```python
from build123d import *

# Parameters (mm, degrees)
SKETCH2_W              = 90
SKETCH2_H              = 90
BOSS_EXTRUDE1_DEPTH    = 300
SKETCH3_W              = 45
SKETCH3_H              = 255
CUT_EXTRUDE1_DEPTH     = 317.425346646
SKETCH4_R              = 25
CRANK_SHAFT_HOLE_DEPTH = 90
SKETCH5_R              = 13
CUT_EXTRUDE3_DEPTH     = 90
CHAMFER1_SIZE          = 3
SKETCH6_R              = 17.5
BOSS_EXTRUDE2_DEPTH    = 30


with BuildPart() as part:
    # Sketch2 → Boss-Extrude1 (new body)
    with BuildSketch(Plane(origin=(0, 0, 0), x_dir=(1, 0, 0), z_dir=(0, 1, 0))):
        Rectangle(SKETCH2_W, SKETCH2_H)
    extrude(amount=BOSS_EXTRUDE1_DEPTH)

    # Sketch3 → Cut-Extrude1 (cut, through all)
    with BuildSketch(Plane(origin=(45, 0, 0), x_dir=(0, 0, -1), z_dir=(1, 0, 0))):
        with Locations((0, 150)):
            Rectangle(SKETCH3_W, SKETCH3_H)
    extrude(amount=-CUT_EXTRUDE1_DEPTH, mode=Mode.SUBTRACT)

    # Sketch4 → Crank shaft hole (cut)
    with BuildSketch(Plane.XY.offset(45)):
        with Locations((0, 170.5)):
            Circle(SKETCH4_R)
    extrude(amount=-CRANK_SHAFT_HOLE_DEPTH, mode=Mode.SUBTRACT)

    # Sketch5 → Cut-Extrude3 (cut)
    with BuildSketch(Plane.XY.offset(45)):
        with Locations((0, 45)):
            Circle(SKETCH5_R)
    extrude(amount=-CUT_EXTRUDE3_DEPTH, mode=Mode.SUBTRACT)

    # Chamfer1
    chamfer1_edges = [part.edges().sort_by_distance(p)[0] for p in [
        (-13, 45, 22.5),
        (-13, 45, -22.5),
    ]]
    chamfer(chamfer1_edges, length=CHAMFER1_SIZE)

    # Sketch6 → Boss-Extrude2 (add)
    with BuildSketch(Plane.XY.offset(45)):
        with Locations(Location((0, 105, 0), (0, 0, 180))):
            Circle(SKETCH6_R)
    boss_extrude2 = extrude(amount=BOSS_EXTRUDE2_DEPTH)

    # Mirror1: Boss-Extrude2 across plane
    add(boss_extrude2.mirror(Plane.XY))


solid = part.part
```
Can you work these out from the model? Positions are in its coordinate system, mm. A direction names the side the tool comes from. Give positions to 0.01 mm unless a question says otherwise; leave off trailing zeros. Write each loop counter-clockwise with the first axis right and the second up, starting at its lowest first coordinate (ties: lowest second). Pieces come first, ordered by that corner, then holes. Notation, with made-up numbers: (5.25, 50) -> (22.25, 50) arc R18 cw to (22.25, 77) -> close; hole circle Ø3 at (11, 66). An arc over 180 degrees is marked (long way). Write item = value, one per line.
(1) Suppose I cut it at C-C on y = 138.5. Write out the boundary of the cut face in (x, z), then the cut area to 3 significant figures.
Worked out:
outline = (-45, -45) -> (45, -45) -> (45, -22.5) -> (-45, -22.5) -> close; (-45, 22.5) -> (45, 22.5) -> (45, 45) -> (-45, 45) -> close
area = 4,050 mm^2
(2) For faces 1 (the face through (7.067, 56.084, -25.354)), 2 (the face through (3.794, 122.084, 59.79)), 3 (the face through (21, 148, -22.5)), 4 (the face through (3.794, 122.084, -59.79)), which set-ups out of +Z, -Z, +X, -X, +Y, -Y let a thin tool reach every point of the face, with its end or its side?
Worked out:
face_1 = none
face_2 = +Z
face_3 = +X, -X
face_4 = -Z
(3) I need wall thicknesses on probe 1 along Y at (x, z) = (0, 38.25); probe 2 along Z at (x, y) = (-32, 236.5); probe 3 along Y at (x, z) = (9, 18). Which ranges of each line are inside material? Lowest first, please. Write a range as from..to.
Worked out:
probe_1 = 0..32, 58..145.5, 195.5..300
probe_2 = -45..-22.5, 22.5..45
probe_3 = 0..22.5, 277.5..300
(4) I'm going to push flat-ended pins straight in: P1, Ø8, axis at x = -21, y = 183.5, coming from the -Z side; P2, Ø1.5, axis at x = 29, y = 42.5, coming from the +Z side. Where does each tip first touch, or does it pass through?
Worked out:
P1 = -45
P2 = 45
(5) Suppose I cut it at B-B on y = 170.5. Write out the boundary of the cut face in (x, z).
Worked out:
outline = (-45, -45) -> (-25, -45) -> (-25, -22.5) -> (-45, -22.5) -> close; (-45, 22.5) -> (-25, 22.5) -> (-25, 45) -> (-45, 45) -> close; (25, -45) -> (45, -45) -> (45, -22.5) -> (25, -22.5) -> close; (25, 22.5) -> (45, 22.5) -> (45, 45) -> (25, 45) -> close
(6) Suppose I cut it at D-D on x = 0. Count the separate pieces of the cut face and the enclosed holes in it, then the cut area to 3 significant figures.
Worked out:
separate_pieces = 4
enclosed_holes = 0
area = 14,200 mm^2
(7) Suppose I cut it at A-A on z = 12.5. Write out the boundary of the cut face in (x, y), then the cut area to 3 significant figures.
Worked out:
outline = (-45, 0) -> (45, 0) -> (45, 22.5) -> (-45, 22.5) -> close; (-45, 277.5) -> (45, 277.5) -> (45, 300) -> (-45, 300) -> close
area = 4,050 mm^2
(8) Thinking about a two-plate mould opening in Y: for faces 5 (the face through (-3.255, 195.287, 33.908)), 6 (the face through (-3.255, 195.287, -33.592)), 7 (the face through (-1, 300, -1)), 8 (the face through (0, 105, 75)), which applies, released by +Y, released by -Y, zero draft, split by the parting line, or undercut?
Worked out:
face_5 = undercut
face_6 = undercut
face_7 = released by +Y
face_8 = zero draft
